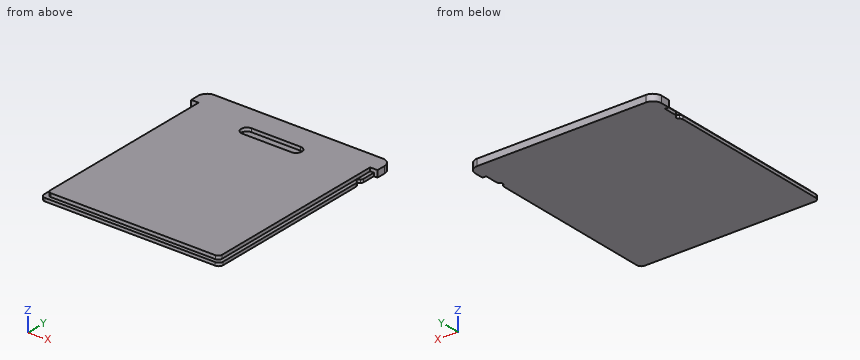
```python
from build123d import *

# Parameters (mm, degrees)
BOSS_EXTRUDE1_DEPTH = 1.8
BOSS_EXTRUDE2_DEPTH = 2
CUT_EXTRUDE1_DEPTH  = 2
SKETCH5_R           = 1.5
CUT_EXTRUDE2_DEPTH  = 1.8
FILLET3_R           = 1.5
FILLET4_R           = 5


with BuildPart() as part:
    # Sketch1 → Boss-Extrude1 (new body)
    with BuildSketch(Plane.XY):
        with BuildLine():
            Line((101.8, 109.8), (103.9, 109.8))
            Line((103.9, 109.8), (103.9, 119.8))
            Line((103.9, 119.8), (-2.1, 119.8))
            Line((-2.1, 119.8), (-2.1, 109.8))
            Line((-2.1, 109.8), (0, 109.8))
            Line((0, 109.8), (0, 2.5))
            ThreePointArc((0, 2.5), (0.732233047, 0.732233047), (2.5, 0))
            Line((2.5, 0), (99.3, 0))
            ThreePointArc((99.3, 0), (101.067766953, 0.732233047), (101.8, 2.5))
            Line((101.8, 2.5), (101.8, 109.8))
        make_face()
    extrude(amount=BOSS_EXTRUDE1_DEPTH)

    # Sketch2 → Boss-Extrude2 (add)
    with BuildSketch(Plane.XY.offset(1.8)):
        with BuildLine():
            Line((2.1, 109.8), (2.1, 4.2))
            ThreePointArc((2.1, 4.2), (2.685786438, 2.785786438), (4.1, 2.2))
            Line((4.1, 2.2), (97.7, 2.2))
            ThreePointArc((97.7, 2.2), (99.114213562, 2.785786438), (99.7, 4.2))
            Line((99.7, 4.2), (99.7, 109.8))
            Line((99.7, 109.8), (103.9, 109.8))
            Line((103.9, 109.8), (103.9, 119.8))
            Line((103.9, 119.8), (-2.1, 119.8))
            Line((-2.1, 119.8), (-2.1, 109.8))
            Line((-2.1, 109.8), (2.1, 109.8))
        make_face()
    extrude(amount=BOSS_EXTRUDE2_DEPTH)

    # Sketch3 → Cut-Extrude1 (cut)
    with BuildSketch(Plane.XY.offset(3.8)):
        with BuildLine():
            Line((35.496856475, 105.630553179), (63.503143525, 105.630553179))
            ThreePointArc((63.503143525, 105.630553179), (66.759688531, 102.374008173), (63.503143525, 99.117463168))
            Line((63.503143525, 99.117463168), (35.496856475, 99.117463168))
            ThreePointArc((35.496856475, 99.117463168), (32.240311469, 102.374008173), (35.496856475, 105.630553179))
        make_face()
    extrude(amount=-CUT_EXTRUDE1_DEPTH, mode=Mode.SUBTRACT)

    # Sketch5 → Cut-Extrude2 (cut)
    with BuildSketch(Plane(origin=(0, 0, 0), x_dir=(-1, 0, 0), z_dir=(0, 0, -1))):
        with Locations((-101.8, 99.8)):
            Circle(SKETCH5_R)
        with Locations((0, 99.8)):
            Circle(SKETCH5_R)
    extrude(amount=-CUT_EXTRUDE2_DEPTH, mode=Mode.SUBTRACT)

    # Fillet3
    fillet3_edges = [part.edges().sort_by_distance(p)[0] for p in [
        (101.8, 101.3, 0.9),
        (101.8, 98.3, 0.9),
        (0, 98.3, 0.9),
        (0, 101.3, 0.9),
    ]]
    fillet(fillet3_edges, radius=FILLET3_R)

    # Fillet4
    fillet4_edges = [part.edges().sort_by_distance(p)[0] for p in [
        (-2.1, 119.8, 1.9),
        (103.9, 119.8, 1.9),
    ]]
    fillet(fillet4_edges, radius=FILLET4_R)


solid = part.part
```
The model under review builds one solid part; all positions refer to its coordinate system, in mm. Round coordinates to 2 decimals unless told otherwise and drop trailing zeros. Loops run counter-clockwise (first coordinate to the right, second up) from the corner with the lowest first, then second, coordinate; pieces in that order, holes last.
Item 1: Clearance check with flat-ended pins moving along their axes: pin 1 Ø3.5 at (x, y) = (42.5, 101) entering from +Z; pin 2 Ø1 at (y, z) = (50, 3) entering from -X; pin 3 Ø2 at (y, z) = (27, 3) entering from +X. State where each tip first meets the part, or that it passes through.
Determined:
pin 1: stops at z = 1.8
pin 2: stops at x = 2.1
pin 3: stops at x = 99.7
Item 2: For line 1 (Y direction, x = 49.5, z = 1.85); line 2 (X direction, y = 49, z = 0.4); line 3 (Y direction, x = 20, z = 3.45), list the stretches that pass through material, from the lowest coordinate up.
Determined:
line 1: y = 2.2 to 99.12, 105.63 to 119.8
line 2: x = 0 to 101.8
line 3: y = 2.2 to 119.8
Item 3: Take a section at A-A (x = 41.5). Write out the cut boundary in (y, z), then the cut area to 3 significant figures.
Determined:
outline: (0, 0) - (119.8, 0) - (119.8, 3.8) - (105.63, 3.8) - (105.63, 1.8) - (99.12, 1.8) - (99.12, 3.8) - (2.2, 3.8) - (2.2, 1.8) - (0, 1.8) - close
area: 438 mm2
Item 4: Take a section at B-B (z = 2.5). Write out the cut boundary in (x, y).
Determined:
outline: (-2.1, 109.8) - (2.1, 109.8) - (2.1, 4.2) arc R2 ccw to (4.1, 2.2) - (97.7, 2.2) arc R2 ccw to (99.7, 4.2) - (99.7, 109.8) - (103.9, 109.8) - (103.9, 114.8) arc R5 ccw to (98.9, 119.8) - (2.9, 119.8) arc R5 ccw to (-2.1, 114.8) - close; hole (35.5, 99.12) - (63.5, 99.12) arc R3.26 ccw to (63.5, 105.63) - (35.5, 105.63) arc R3.26 ccw to start
Item 5: Take a section at C-C (y = 12.5). Write out the cut boundary in (x, z), then the cut area to 3 significant figures.
Determined:
outline: (0, 0) - (101.8, 0) - (101.8, 1.8) - (99.7, 1.8) - (99.7, 3.8) - (2.1, 3.8) - (2.1, 1.8) - (0, 1.8) - close
area: 378 mm2
